Design review of the part built by this model. Coordinates are the model's own, in mm. A direction names the side the tool comes from. Give positions to 0.01 mm unless a question says otherwise; leave off trailing zeros. Loops run counter-clockwise (first coordinate to the right, second up) from the corner with the lowest first, then second, coordinate; pieces in that order, holes last.
from build123d import *

# Parameters (mm, degrees)
EXTRUDE_1_DEPTH              = 8
SKETCH_2_W                   = 150
SKETCH_2_H                   = 8
EXTRUDE_2_DEPTH              = 20
SKETCH_3_W                   = 20
SKETCH_3_H                   = 8
EXTRUDE_3_DEPTH              = 20
SKETCH_4_W                   = 20
SKETCH_4_H                   = 8
EXTRUDE_4_DEPTH              = 20
SKETCH_5_W                   = 8
SKETCH_5_H                   = 40
EXTRUDE_5_DEPTH              = 20
CUT_EXTRUDE_1_DEPTH          = 20
EXTRUDE_6_DEPTH              = 40
HOLE_WIZARD_2_D              = 3.2
HOLE_WIZARD_2_DEPTH          = 8
HOLE_WIZARD_2_CSINK_D        = 5.6
HOLE_WIZARD_2_CSINK_ANGLE    = 82
HOLE_WIZARD_2_TIP            = 0.96137699
HOLE_WIZARD_M4_1_D           = 4.8
HOLE_WIZARD_M4_1_DEPTH       = 8.95
HOLE_WIZARD_M4_1_CSINK_D     = 9.4
HOLE_WIZARD_M4_1_CSINK_ANGLE = 90
SKETCH_17_R                  = 2.6
CUT_EXTRUDE_3_DEPTH          = 40
SKETCH_22_R                  = 2.25
CUT_EXTRUDE_4_DEPTH          = 74.15
SKETCH_24_W                  = 60
SKETCH_24_H                  = 0.68
CUT_EXTRUDE_5_DEPTH          = 40
SKETCH_29_W                  = 44
SKETCH_29_H                  = 0.5
CUT_EXTRUDE_10_DEPTH         = 81


with BuildPart() as part:
    # 草图1 → 凸台-拉伸1 (new body)
    with BuildSketch(Plane.XY):
        Polygon((-23.56557377, -33.278688525), (51.43442623, -33.278688525), (88.93442623, 6.721311475), (88.93442623, 23.721311475), (58.93442623, 46.721311475), (-31.06557377, 46.721311475), (-61.06557377, 23.721311475), (-61.06557377, 6.721311475), align=None)
    extrude(amount=EXTRUDE_1_DEPTH)

    # 草图2 → 凸台-拉伸2 (add)
    with BuildSketch(Plane.XY.offset(8)):
        with Locations((13.93442623, 10.721311475)):
            Rectangle(SKETCH_2_W, SKETCH_2_H)
    extrude(amount=EXTRUDE_2_DEPTH)

    # 草图3 → 凸台-拉伸3 (add)
    with BuildSketch(Plane(origin=(88.93442623, 0, 0), x_dir=(0, 0, -1), z_dir=(1, 0, 0))):
        with Locations((-18, 10.721311475)):
            Rectangle(SKETCH_3_W, SKETCH_3_H)
    extrude(amount=EXTRUDE_3_DEPTH)

    # 草图4 → 凸台-拉伸4 (add)
    with BuildSketch(Plane.ZY.offset(61.06557377)):
        with Locations((18, 10.721311475)):
            Rectangle(SKETCH_4_W, SKETCH_4_H)
    extrude(amount=EXTRUDE_4_DEPTH)

    # 草图5 → 凸台-拉伸5 (add)
    with BuildSketch(Plane.XY.offset(8)):
        with Locations((13.93442623, -13.278688525)):
            Rectangle(SKETCH_5_W, SKETCH_5_H)
    extrude(amount=EXTRUDE_5_DEPTH)

    # 草图6 → 切除-拉伸1 (cut)
    with BuildSketch(Plane(origin=(17.93442623, 0, 0), x_dir=(0, 0, -1), z_dir=(1, 0, 0))):
        Polygon((-18, -33.278688525), (-28, 0.111311475), (-28, -33.278688525), align=None)
    extrude(amount=-CUT_EXTRUDE_1_DEPTH, mode=Mode.SUBTRACT)

    # 草图7 → 凸台-拉伸6 (add)
    with BuildSketch(Plane(origin=(0, 46.721311475, 0), x_dir=(1, 0, 0), z_dir=(0, 1, 0))):
        Polygon((-8.06557377, 36.2), (35.93442623, 36.2), (35.93442623, 0), (43.93442623, 0), (43.93442623, 45.15), (-16.06557377, 45.15), (-16.06557377, 0), (-8.06557377, 0), align=None)
    extrude(amount=-EXTRUDE_6_DEPTH)

    # 孔2
    with Locations(Plane(origin=(1.420779952, 23.721311475, 8), x_dir=(1, 0, 0), z_dir=(0, 0, 1))):
        with Locations((0, 0), (25.013646278, 0), (25.013646278, -25), (0.013646278, -25)):
            CounterSinkHole(HOLE_WIZARD_2_D / 2, HOLE_WIZARD_2_CSINK_D / 2, depth=HOLE_WIZARD_2_DEPTH, counter_sink_angle=HOLE_WIZARD_2_CSINK_ANGLE)
            with Locations((0, 0, -(HOLE_WIZARD_2_DEPTH + HOLE_WIZARD_2_TIP / 2))):  # 118° drill point
                Cone(0, HOLE_WIZARD_2_D / 2, HOLE_WIZARD_2_TIP, mode=Mode.SUBTRACT)

    # M4 平头机械螺钉的锥形沉头孔1
    with Locations(Plane(origin=(1.93442623, 16.721311475, -36.2), x_dir=(1, 0, 0), z_dir=(0, 0, 1))):
        with Locations((0, 0), (24, 0), (24, 20), (0, 20)):
            CounterSinkHole(HOLE_WIZARD_M4_1_D / 2, HOLE_WIZARD_M4_1_CSINK_D / 2, depth=HOLE_WIZARD_M4_1_DEPTH, counter_sink_angle=HOLE_WIZARD_M4_1_CSINK_ANGLE)

    # 草图17 → 切除-拉伸3 (cut)
    with BuildSketch(Plane(origin=(0, 14.721311475, 0), x_dir=(1, 0, 0), z_dir=(0, 1, 0))):
        with Locations((85.18442623, -18)):
            Circle(SKETCH_17_R)
        with Locations((37.311975267, -18)):
            Circle(SKETCH_17_R)
        with Locations((-9.81557377, -18)):
            Circle(SKETCH_17_R)
        with Locations((-57.31557377, -18.235938013)):
            Circle(SKETCH_17_R)
    extrude(amount=-CUT_EXTRUDE_3_DEPTH, mode=Mode.SUBTRACT)

    # 草图22 → 切除-拉伸4 (cut, through all)
    with BuildSketch(Plane(origin=(0, 0, -45.15), x_dir=(-1, 0, 0), z_dir=(0, 0, -1))):
        with Locations((-25.93442623, 36.721311475)):
            Circle(SKETCH_22_R)
        with Locations((-1.93442623, 36.721311475)):
            Circle(SKETCH_22_R)
        with Locations((-1.93442623, 16.721311475)):
            Circle(SKETCH_22_R)
        with Locations((-25.93442623, 16.721311475)):
            Circle(SKETCH_22_R)
    extrude(amount=-CUT_EXTRUDE_4_DEPTH, mode=Mode.SUBTRACT)

    # 草图24 → 切除-拉伸5 (cut)
    with BuildSketch(Plane(origin=(0, 46.721311475, 0), x_dir=(1, 0, 0), z_dir=(0, 1, 0))):
        with Locations((13.93442623, 44.81)):
            Rectangle(SKETCH_24_W, SKETCH_24_H)
    extrude(amount=-CUT_EXTRUDE_5_DEPTH, mode=Mode.SUBTRACT)

    # 草图29 → 切除-拉伸10 (cut, through all)
    with BuildSketch(Plane(origin=(0, 46.721311475, 0), x_dir=(1, 0, 0), z_dir=(0, 1, 0))):
        with Locations((13.93442623, 36.45)):
            Rectangle(SKETCH_29_W, SKETCH_29_H)
    extrude(amount=-CUT_EXTRUDE_10_DEPTH, mode=Mode.SUBTRACT)


solid = part.part
Q1. Take a section at A-A (z = -32.5). Give the boundary of the cut face in (x, y), plus the area to 3 significant figures.
Results:
outline: (-16.07, 6.72) - (-8.07, 6.72) - (-8.07, 46.72) - (-16.07, 46.72) - close; (35.93, 6.72) - (43.93, 6.72) - (43.93, 46.72) - (35.93, 46.72) - close
area: 640 mm2
Q2. Draft analysis for pull direction X (two halves, no side actions). For faces 1 (the face through (-71, 11, 8)), 2 (the face through (-12.413, 10.777, 17.886)), 3 (the face through (108.934, 11, 18)), state which applies: pulls with the +X half, pulls with the -X half, needs draft (parallel to the pull), parting line crosses it, or undercut.
Results:
face 1: needs draft
face 2: undercut
face 3: pulls with the +X half
Q3. Wall thickness on line 1 (X direction, y = 40.5, z = -7.5); line 2 (X direction, y = 38, z = 5); line 3 (Y direction, x = -17.5, z = 20): over which ranges is each line inside the solid? List them lowest first.
Results:
line 1: x = -16.07 to -8.07, 35.93 to 43.93
line 2: x = -42.44 to 0.08, 3.79 to 24.08, 27.79 to 70.31
line 3: y = 6.72 to 14.72
Q4. Tool access review of faces 4 (the face through (-16.066, 27, -23)), 5 (the face through (69, 14.721, 18)), 6 (the face through (35.934, 27, -19)), 7 (the face through (0.83, 14.59, -41.53)), 8 (the face through (17.934, -9, 16)): name each direction out of +Z, -Z, +X, -X, +Y, -Y from which nothing blocks a thin tool from reaching the whole face with its end or side.
Results:
face 4: -Z, -X, +Y, -Y
face 5: +Z, +X, -X, +Y
face 6: +Y, -Y
face 7: -Z
face 8: +Z, +X, -Y
Q5. Insertion check: pin 1 (7 mm diameter, centred on x = 1.93, y = 36.72, fed in from +Z); pin 2 (5 mm diameter, centred on y = -19, z = 9.5, fed in from +X); pin 3 (2.5 mm diameter, centred on x = 25.93, y = 36.72, fed in from +Z); pin 4 (12 mm diameter, centred on y = 24, z = -11.5, fed in from +X). Each pin has a flat end and moves straight along its axis. Give the tip position at first contact, or say it passes through.
Results:
pin 1: stops at z = 8
pin 2: stops at x = 66.7
pin 3: passes through
pin 4: stops at x = 43.93
Q6. Take a section at C-C (y = -19.5). Give the boundary of the cut face in (x, z).
Results:
outline: (-36.48, 0) - (64.35, 0) - (64.35, 8) - (17.93, 8) - (17.93, 22.13) - (9.93, 22.13) - (9.93, 8) - (-36.48, 8) - close
Q7. Take a section at B-B (x = -56.5). Give the boundary of the cut face in (y, z).
Results:
outline: (1.85, 0) - (27.22, 0) - (27.22, 8) - (14.72, 8) - (14.72, 15.77) - (6.72, 15.77) - (6.72, 8) - (1.85, 8) - close; (6.72, 20.7) - (14.72, 20.7) - (14.72, 28) - (6.72, 28) - close
Q8. Take a section at D-D (z = 13.5). Give the boundary of the cut face in (x, y).
Results:
outline: (-81.07, 6.72) - (9.93, 6.72) - (9.93, -33.28) - (17.93, -33.28) - (17.93, 6.72) - (108.93, 6.72) - (108.93, 14.72) - (26.97, 14.72) arc R2.25 cw to (24.9, 14.72) - (2.97, 14.72) arc R2.25 cw to (0.9, 14.72) - (-81.07, 14.72) - close
